from build123d import *

# Parameters (mm, degrees)
SKETCH1_W           = 17.78
SKETCH1_H           = 17.78
BOSS_EXTRUDE1_DEPTH = 1
SKETCH2_R           = 3.5
BOSS_EXTRUDE2_DEPTH = 2
SKETCH3_W           = 5.587821929
SKETCH3_H           = 2.090408203
SKETCH3_W_2         = 2.613010254
SKETCH3_H_2         = 5.065219877
BOSS_EXTRUDE3_DEPTH = 3
SKETCH4_W           = 8.382
SKETCH4_H           = 2.54
BOSS_EXTRUDE4_DEPTH = 3
SKETCH5_W           = 0.4064
SKETCH5_H           = 0.6096
BOSS_EXTRUDE5_DEPTH = 3


with BuildPart() as part:
    # Sketch1 → Boss-Extrude1 (new body)
    with BuildSketch(Plane(origin=(0, 0, 0), x_dir=(1, 0, 0), z_dir=(0, 1, 0))):
        Rectangle(SKETCH1_W, SKETCH1_H)
    extrude(amount=BOSS_EXTRUDE1_DEPTH)

    # Sketch2 → Boss-Extrude2 (add)
    with BuildSketch(Plane(origin=(0, 1, 0), x_dir=(1, 0, 0), z_dir=(0, 1, 0))):
        with Locations(Location((-3.2361127, 2.643160373, 0), (0, 0, 90))):
            Circle(SKETCH2_R)
    extrude(amount=BOSS_EXTRUDE2_DEPTH)

    # Sketch3 → Boss-Extrude3 (add)
    with BuildSketch(Plane(origin=(0, 1, 0), x_dir=(1, 0, 0), z_dir=(0, 1, 0))):
        with Locations((5.165720273, -2.16075848)):
            Rectangle(SKETCH3_W, SKETCH3_H)
        with Locations((3.015011832, 2.68336053)):
            Rectangle(SKETCH3_W_2, SKETCH3_H_2)
    extrude(amount=BOSS_EXTRUDE3_DEPTH)

    # Sketch4 → Boss-Extrude4 (add)
    with BuildSketch(Plane(origin=(0, 1, 0), x_dir=(1, 0, 0), z_dir=(0, 1, 0))):
        with Locations((0, -7.62)):
            Rectangle(SKETCH4_W, SKETCH4_H)
    extrude(amount=BOSS_EXTRUDE4_DEPTH)

    # Sketch5 → Boss-Extrude5 (add)
    with BuildSketch(Plane.XY.offset(8.89)):
        with Locations((-2.54, 3.6952)):
            Rectangle(SKETCH5_W, SKETCH5_H)
        with Locations((0, 3.6952)):
            Rectangle(SKETCH5_W, SKETCH5_H)
        with Locations((2.54, 3.6952)):
            Rectangle(SKETCH5_W, SKETCH5_H)
    extrude(amount=BOSS_EXTRUDE5_DEPTH)


solid = part.part
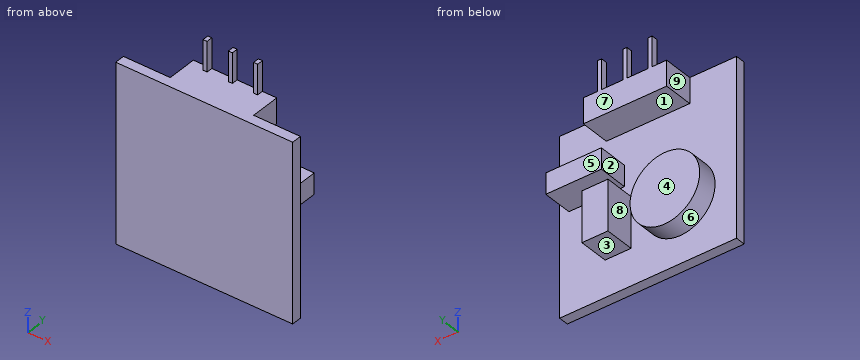
Design review of the part built by this model. Coordinates are the model's own, in mm. Face numbers are marked on the shaded views. A direction names the side the tool comes from. Round coordinates to 2 decimals unless told otherwise and drop trailing zeros. Write each loop counter-clockwise with the first axis right and the second up, starting at its lowest first coordinate (ties: lowest second). Pieces come first, ordered by that corner, then holes. Notation, with made-up numbers: M -31.75,22 L -0.75,22 A13 cw -0.75,43 Z; hole C 29.25,78.25 d7. An arc over 180 degrees is marked long. One line per item, written item: value. Start each with the question number.
1. Clearance check with flat-ended pins moving along their axes: P1, Ø2, axis at y = 3, z = 8, coming from the -X side; P2, Ø7.5, axis at x = -4.5, z = -2.5, coming from the +Y side; P3, Ø0.9, axis at y = 2, z = -3.5, coming from the +X side. State where each tip first meets the part, or that it passes through.
2. Take a section at A-A on x = 0.5. State the section outline as (y, z) points.
3. Take a section at C-C on z = -4. State the section outline as (x, y) points.
4. Draft analysis for pull direction X (two halves, no side actions). For the marked faces 6, 7, 8 and 9, state which applies: pulls with the +X half, pulls with the -X half, needs draft (parallel to the pull), parting line crosses it, or undercut.
5. Take a section at D-D on y = 0.55. State the section outline as (x, z) points.
6. For the marked faces 1, 2, 3, 4 and 5, list the 3-axis set-ups (+Z, -Z, +X, -X, +Y, -Y) from which the entire face can be reached by the end or side of a thin tool; tool diameter is ignored.
7. Take a section at B-B on y = 2.55. State the section outline as (x, z) points.
8. To check wall thickness, follow probe 1 along Z at (x, y) = (3.5, 2); probe 2 along X at (y, z) = (1.55, -2.5); probe 3 along Z at (x, y) = (-4, 0.8). State the ranges of each line that lie inside material, in increasing order. Write a range as from..to.
Computed:
1. P1: stops at x = -4.19
1. P2: stops at y = 3
1. P3: stops at x = 4.32
2. outline: M 0,-8.89 L 1,-8.89 L 1,6.35 L 4,6.35 L 4,8.89 L 0,8.89 Z
3. outline: M -8.89,0 L 8.89,0 L 8.89,1 L 4.32,1 L 4.32,4 L 1.71,4 L 1.71,1 L -0.01,1 L -0.01,3 L -6.46,3 L -6.46,1 L -8.89,1 Z
4. face 6: undercut
4. face 7: needs draft
4. face 8: undercut
4. face 9: pulls with the -X half
5. outline: M -8.89,-8.89 L 8.89,-8.89 L 8.89,8.89 L -8.89,8.89 Z
6. face 1: +X, -X, +Y
6. face 2: -X, +Y
6. face 3: -Z, +X, +Y
6. face 4: -Z, -X, +Y
6. face 5: +Z, -Z, +X, -X, +Y
7. outline: C -3.24,-2.64 d7; M -4.19,6.35 L 4.19,6.35 L 4.19,8.89 L -4.19,8.89 Z; M 1.71,-5.22 L 4.32,-5.22 L 4.32,-0.15 L 1.71,-0.15 Z; M 2.37,1.12 L 7.96,1.12 L 7.96,3.21 L 2.37,3.21 Z
8. probe 1: z = -5.22..-0.15, 1.12..3.21, 6.35..8.89
8. probe 2: x = -6.73..0.26, 1.71..4.32
8. probe 3: z = -8.89..8.89
